Input: part model. Units: mm. Frame: model coordinates. A direction names the side the tool comes from. Coordinates: 2 decimals unless noted, no trailing zeros. Order: outer loops, then holes, each group sorted by start corner. A loop starts at its lowest first (then second) coordinate and runs counter-clockwise, first axis right, second up. Notation, with made-up numbers: (12, -11.75) - (56, -11.75) arc R17 cw to (56, 14.25) - close; hole circle Ø11 at (19, -12). An arc over 180 degrees is marked (long way). Answer as CSV lines item,"result". Start each with the question number.
Item 1: Material intervals for line 1 along Z through (x, y) = (37, 27); line 2 along X through (y, z) = (22, 25); line 3 along Z through (x, y) = (53, 52), sorted ascending.
Item 2: Section C-C (x = 37.5). Output: boundary loops of the cut face in (y, z).
Item 3: Section A-A (z = 25). Output: boundary loops of the cut face in (x, y).
Item 4: Access query for faces 1 (the flat face through (38, 30, 10)), 2 (the flat face through (75, 30, 45)), 3 (the flat face through (51, 0, 25)). Directions: +Z, -Z, +X, -X, +Y, -Y. A direction counts if a zero-diameter tool reaches every point of the face in a straight line with its end or side. Return the directions, or none.
Item 5: Draft query along X for faces 4 (the flat face through (85, 30, 25)), 5 (the flat face through (75, 30, 5)), 6 (the flat face through (80, 30, 50)), 7 (the cylindrical face through (47.04, 30.42, 22)). Return one class per face: +X half, -X half, draft (parallel to the pull), parting line (faces both ways), or undercut.
Item 6: Section D-D (x = 72). Output: boundary loops of the cut face in (y, z).
Item 7: First-contact query: pin 1 (3 mm diameter, centred on x = 52.5, y = 37, fed in from +Z); pin 2 (1.5 mm diameter, centred on x = 36, y = 46.5, fed in from -Z); pin 3 (2 mm diameter, centred on y = 16.5, z = 43.5, fed in from -X). Flat tips, straight axial feed; report the tip coordinate or a pass-through.
Item 8: Section B-B (y = 8.5). Output: boundary loops of the cut face in (x, z).
Autodesk Inventor part; units mm, degrees
ref_plane "YZ Plane" through (0, 0, 0) normal (1, 0, 0) x (0, 1, 0)
ref_plane "XZ Plane" through (0, 0, 0) normal (0, 1, 0) x (-1, 0, 0)
ref_plane "XY Plane" through (0, 0, 0) normal (0, 0, 1) x (1, 0, 0)
sketch "Boceto1" plane through (0, 0, 0) normal (0, 0, 1) x (1, 0, 0)
  line L0 (0, 0) -> (85, 0)
  line L1 (85, 0) -> (85, 60)
  line L2 (0, 60) -> (0, 0)
  line L3 (0, 60) -> (85, 60)
  dimension "d0" = 85
  dimension "d1" = 60
extrude "Extrusión1" add sketch "Boceto1" along normal blind 50
sketch "Boceto3" plane through (0, 0, 50) normal (0, 0, 1) x (1, 0, 0)
  point P0 (0, 0)
ref_plane "Plano de trabajo3" through (0, 60, 50) normal (0, 0, 1) x (1, 0, 0)
sketch "Boceto4" plane through (0, 60, 50) normal (0, 0, 1) x (1, 0, 0)
  line L0 (0, -60) -> (85, -60)
  line L1 (0, -60) -> (75, -60)
  line L2 (75, -60) -> (75, 0)
  line L3 (75, 0) -> (0, 0)
  line L4 (0, 0) -> (0, -60)
  line L5 (0, 0) -> (0, -60)
  dimension "d7" = 75
  dimension "d8" = 60
extrude "Extrusión2" cut sketch "Boceto4" against normal blind 10
sketch "Boceto5" plane through (0, 0, 0) normal (0, 0, -1) x (-1, 0, 0)
  line L0 (0, 0) -> (-85, 0)
  line L1 (0, 0) -> (-75, 0)
  line L2 (-75, 0) -> (-75, 60)
  line L3 (-85, 60) -> (0, 60)
  line L4 (-75, 60) -> (0, 60)
  line L5 (0, 60) -> (0, 0)
  line L6 (0, 60) -> (0, 0)
  dimension "d11" = 75
  dimension "d12" = 60
extrude "Extrusión3" cut sketch "Boceto5" against normal blind 10
ref_plane "Plano de trabajo5" through (85, 60, 50) normal (0, 1, 0) x (1, 0, 0)
sketch "Boceto6" plane through (85, 60, 50) normal (0, 1, 0) x (1, 0, 0)
  line L0 (-85, 10) -> (-10, 10)
  line L1 (-10, 40) -> (-85, 40)
  circle A0 centre (-47.5, 25) radius 10
  point P0 (-85, 50)
  dimension "d15" = 20
extrude "Extrusión4" cut sketch "Boceto6" against normal through all
thread "Rosca1"
properties part number "SoporteHerramienta"
Determined:
1,line 1,"z = 10 to 15.01, 34.99 to 40"
1,line 2,"x = 0 to 27.5, 47.5 to 85"
1,line 3,"z = 10 to 40"
2,outline,"(0, 10) - (60, 10) - (60, 15) - (0, 15) - close; (0, 35) - (60, 35) - (60, 40) - (0, 40) - close"
3,outline,"(0, 0) - (27.5, 0) - (27.5, 60) - (0, 60) - close; (47.5, 0) - (85, 0) - (85, 60) - (47.5, 60) - close"
4,face 1,"-Z, -X, +Y, -Y"
4,face 2,"+Z, -X, +Y, -Y"
4,face 3,"+Z, -Z, +X, -X, -Y"
5,face 4,"+X half"
5,face 5,"-X half"
5,face 6,"draft"
5,face 7,"undercut"
6,outline,"(0, 10) - (60, 10) - (60, 40) - (0, 40) - close"
7,pin 1,"stops at z = 40"
7,pin 2,"stops at z = 10"
7,pin 3,"stops at x = 75"
8,outline,"(0, 10) - (75, 10) - (75, 0) - (85, 0) - (85, 50) - (75, 50) - (75, 40) - (0, 40) - close; hole circle Ø20 at (37.5, 25)"
